Build history of the part. All positions in model axes, mm. Face numbers are marked on the shaded views. Give positions to 0.01 mm unless a question says otherwise; leave off trailing zeros. Write each loop counter-clockwise with the first axis right and the second up, starting at its lowest first coordinate (ties: lowest second). Pieces come first, ordered by that corner, then holes.
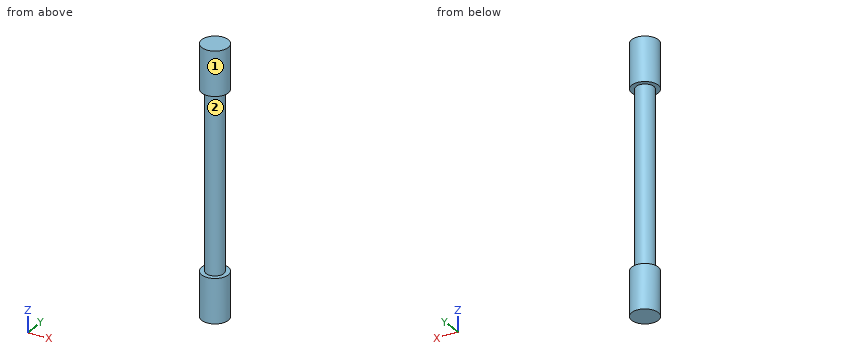
from build123d import *

# Parameters (mm, degrees)
BOSS_EXTRUDE1_DEPTH      = 20
BOSS_EXTRUDE1_DEPTH_BACK = 20
SKETCH1_R                = 2
SKETCH2_R                = 3
BOSS_EXTRUDE2_DEPTH      = 10


with BuildPart() as part:
    # Sketch1 → Boss-Extrude1 (new, two sides: drawn at the far end of the back side and taken through both)
    with BuildSketch(Plane.XY.offset(-BOSS_EXTRUDE1_DEPTH_BACK)):
        Circle(SKETCH1_R)
    extrude(amount=BOSS_EXTRUDE1_DEPTH + BOSS_EXTRUDE1_DEPTH_BACK)

    # Sketch2 → Boss-Extrude2 (add)
    with BuildSketch(Plane.XY.offset(20)):
        Circle(SKETCH2_R)
    boss_extrude2 = extrude(amount=BOSS_EXTRUDE2_DEPTH)

    # Mirror1: Boss-Extrude2 across plane
    add(boss_extrude2.mirror(Plane.XY))


solid = part.part
1. Mould opens along Z. For the marked faces 1 and 2 say: pulls with the +Z half, pulls with the -Z half, needs draft (parallel to the pull), parting line crosses it, or undercut.
2. Saw through at A-A on y = 0. Give the cut face in (x, z).
3. Saw through at C-C on z = 0. Give the cut face in (x, y).
4. Drop flat-ended pins along their axis: pin 1 (1 mm diameter, centred on x = 1.5, z = -15.5, fed in from -Y); pin 2 (1.5 mm diameter, centred on x = 0.5, z = -1.5, fed in from -Y); pin 3 (2 mm diameter, centred on x = 1.5, z = 6.5, fed in from +Y). Give the stop position or say it passes through.
5. Drill centre lines: line 1 along Z through (x, y) = (2.5, -1.45); line 2 along Y through (x, z) = (-0.25, 21.5); line 3 along Y through (x, z) = (0, 6). Where is each one in solid material? Low to high.
Outcome:
1. face 1: needs draft
1. face 2: undercut
2. outline: (-3, -30) - (3, -30) - (3, -20) - (2, -20) - (2, 20) - (3, 20) - (3, 30) - (-3, 30) - (-3, 20) - (-2, 20) - (-2, -20) - (-3, -20) - close
3. outline: circle Ø4 at (0, 0)
4. pin 1: stops at y = -1.73
4. pin 2: stops at y = -2
4. pin 3: stops at y = 1.94
5. line 1: z = -30 to -20, 20 to 30
5. line 2: y = -2.99 to 2.99
5. line 3: y = -2 to 2
